Geometry check sheet. Reference: the model listing, model coordinates, mm. Face numbers are marked on the shaded views. A direction names the side the tool comes from. Give positions to 0.01 mm unless a question says otherwise; leave off trailing zeros. Order: outer loops, then holes, each group sorted by start corner. A loop starts at its lowest first (then second) coordinate and runs counter-clockwise, first axis right, second up.
Autodesk Fusion 360 part; units mm, degrees
sketch "Sketch1" plane through (0, 0, 0) normal (0, 1, 0) x (1, 0, 0)
  line L0 (0, 0) -> (10, 0)
  line L1 (5, 0) -> (5, 10)
  line L2 (0, 0) -> (0, 15)
  line L3 (0, 15) -> (10, 15)
  line L4 (10, 15) -> (10, 0)
  circle A0 centre (5, 10) radius 1.5
  dimension "d1" = 3
extrude "Extrude1" add sketch "Sketch1" along normal blind 5
sketch "Sketch2" plane through (0, 0, 0) normal (0, 0, 1) x (1, 0, 0)
  line L0 (0, 0) -> (10, 0)
  line L1 (10, 0) -> (10, 5)
  line L2 (10, 5) -> (0, 5)
  line L3 (0, 5) -> (0, 0)
  line L4 (5, 0) -> (5, 10)
  line L5 (0, 5) -> (0, 15)
  line L6 (0, 15) -> (10, 15)
  line L7 (10, 15) -> (10, 5)
  circle A0 centre (5, 10) radius 1.5
  dimension "d4" = 10
  dimension "d5" = 3
extrude "Extrude2" add sketch "Sketch2" against normal blind 5 contours L2 L5 L6 L7
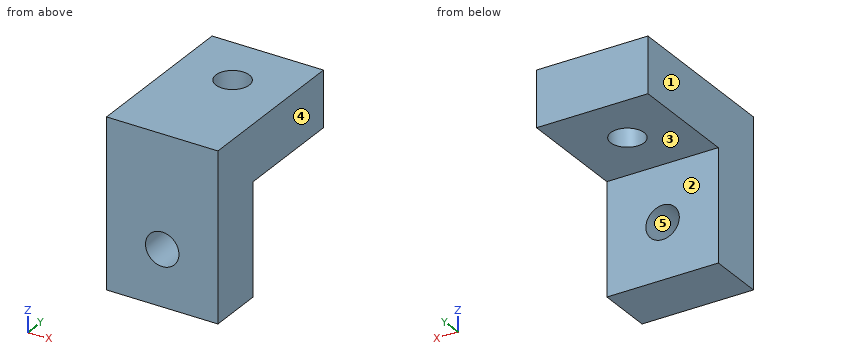
Item 1: Sectioned sample at D-D (x = 1). Enter the section's corners in (y, z).
Reported:
outline: (0, -15) - (5, -15) - (5, -5) - (15, -5) - (15, 0) - (0, 0) - close
Item 2: Sectioned sample at C-C (x = 5). Enter the section's corners in (y, z).
Reported:
outline: (0, -15) - (5, -15) - (5, -11.5) - (0, -11.5) - close; (0, -8.5) - (5, -8.5) - (5, -5) - (8.5, -5) - (8.5, 0) - (0, 0) - close; (11.5, -5) - (15, -5) - (15, 0) - (11.5, 0) - close
Item 3: Sectioned sample at A-A (y = 10). Enter the section's corners in (x, z).
Reported:
outline: (0, -5) - (3.5, -5) - (3.5, 0) - (0, 0) - close; (6.5, -5) - (10, -5) - (10, 0) - (6.5, 0) - close
Item 4: Gauge pin test, flat ends, axial feed: pin 1 (5 mm diameter, centred on x = 4, y = 8.5, fed in from -Z); pin 2 (5 mm diameter, centred on x = 5, z = -10, fed in from +Y). Record the tip position at first contact, or that the pin passes through.
Reported:
pin 1: stops at z = -5
pin 2: stops at y = 5
Item 5: Draft check along X on the marked faces 3, 4 and 5. Enter one of: released by +X, released by -X, zero draft, split by the parting line, or undercut.
Reported:
face 3: zero draft
face 4: released by +X
face 5: undercut
Item 6: Scan lines: L1, parallel to X at y = 1.6, z = -10; L2, parallel to Z at x = 5, y = 2.8; L3, parallel to Y at x = 5, z = -1.2. Record each from-to range of solid material in increasing order.
Reported:
L1: x = 0 to 3.5, 6.5 to 10
L2: z = -15 to -11.5, -8.5 to 0
L3: y = 0 to 8.5, 11.5 to 15
Item 7: Set-up check for the marked faces 1 and 2: record each of +Z, -Z, +X, -X, +Y, -Y from which the full face is reachable in a straight line by a thin tool's end or side.
Reported:
face 1: +Z, -Z, -X, +Y, -Y
face 2: -Z, +X, -X, +Y
Item 8: Sectioned sample at B-B (z = -10). Enter the section's corners in (x, y).
Reported:
outline: (0, 0) - (3.5, 0) - (3.5, 5) - (0, 5) - close; (6.5, 0) - (10, 0) - (10, 5) - (6.5, 5) - close
